The listing builds one solid part. Answer for the finished solid, in the listing's coordinates (mm). Face numbers are marked on the shaded views. A direction names the side the tool comes from. Round coordinates to 2 decimals unless told otherwise and drop trailing zeros. Order: outer loops, then holes, each group sorted by start corner. A loop starts at its lowest first (then second) coordinate and runs counter-clockwise, first axis right, second up. Notation, with made-up numbers: (-32, 86.5) - (27, 86.5) arc R18 ccw to (27, 101.5) - close; hole circle Ø3 at (69.25, 83.5). An arc over 180 degrees is marked (long way). Use CSV: the item, a comma, the result in double quotes. Start each with the question number.
Item 1: Flat-ended cylindrical pins translate along their axes: P1, Ø24, axis at x = 1, y = -3, coming from the +Z side; P2, Ø8, axis at x = 7, y = 8.5, coming from the +Z side; P3, Ø3, axis at y = 2, z = 14.5, coming from the +X side. Find the tip coordinate at first contact, or state that the pin passes through.
Item 2: For the marked faces 4 and 5, determine the directions among +Z, -Z, +X, -X, +Y, -Y from which every point of the face is accessible in a straight line to the end or side of a thin tool.
Item 3: Straight lines are drawn through the part: line 1 along Y through (x, z) = (0, 42.45); line 2 along Z through (x, y) = (2.5, 7); line 3 along Z through (x, y) = (-12.5, -3). For each, find the intervals that lie inside material, in ascending order. Write a range as [from, to].
Item 4: Find section D-D, the plane z = 50. Give the vertices of the cut face in (x, y).
Item 5: Determine the mould class of the marked faces 1, 2 and 3 for opening direction Z: +Z half, -Z half, draft (parallel to the pull), parting line (faces both ways), or undercut.
Solid Edge part; units mm, degrees
sketch "Sketch1" plane through (0, 0, 0) normal (0, 0, 1) x (1, 0, 0)
  line L0 (-20.5, -20.5) -> (20.5, -20.5)
  line L1 (20.5, -20.5) -> (20.5, 20.5)
  line L2 (20.5, 20.5) -> (-20.5, 20.5)
  line L3 (-20.5, 20.5) -> (-20.5, -20.5)
extrude "ProtrusiónExtruida_1" add sketch "Sketch1" along normal blind 41
sketch "Sketch2" plane through (0, 0, 41) normal (0, 0, 1) x (1, 0, 0)
  circle A0 centre (0, 0) radius 9
  circle A1 centre (0, 0) radius 11
extrude "ProtrusiónExtruida_2" add sketch "Sketch2" along normal blind 2
sketch "Sketch3" plane through (0, 0, 41) normal (0, 0, 1) x (1, 0, 0)
  circle A0 centre (0, 0) radius 2.5
extrude "ProtrusiónExtruida_3" add sketch "Sketch3" along normal blind 20
sketch "Sketch4" plane through (0, 0, 0) normal (0, -1, 0) x (1, 0, 0)
  line L0 (2.5, 58) -> (8, 58)
  line L1 (8, 58) -> (8, 57)
  line L2 (8, 57) -> (6, 57)
  line L3 (6, 57) -> (6, 45)
  line L4 (6, 45) -> (2.5, 45)
  line L5 (2.5, 45) -> (2.5, 58)
revolve "RevolvedProtrusion1" add sketch "Sketch4" angle 360 about axis through (0, 0, -54) along (0, 0, 1)
sketch "Sketch5" plane through (20.5, 0, 20.5) normal (1, 0, 0) x (0, 1, 0)
  line L0 (20.5, -11.5) -> (20.5, 13)
  line L1 (20.5, 13) -> (20.49, 13)
  line L2 (20.49, 13) -> (20.49, -11.5)
  line L3 (20.49, -11.5) -> (20.5, -11.5)
extrude "Cutout1" cut sketch "Sketch5" against normal up to next
sketch "Sketch6" plane through (0, 20.49, 21.25) normal (0, 1, 0) x (-1, 0, 0)
  line L0 (20.5, 12.25) -> (20.5, -12.25)
  line L1 (20.49, -12.25) -> (20.5, -12.25)
  line L2 (20.49, 12.25) -> (20.49, -12.25)
  line L3 (20.5, 12.25) -> (20.49, 12.25)
extrude "Cutout2" cut sketch "Sketch6" against normal up to next
sketch "Sketch7" plane through (-20.49, -0.005, 21.25) normal (-1, 0, 0) x (0, -1, 0)
  line L0 (20.485, 12.25) -> (20.485, -12.25)
  line L1 (20.485, -12.25) -> (20.495, -12.25)
  line L2 (20.495, -12.25) -> (20.495, 12.25)
  line L3 (20.495, 12.25) -> (20.485, 12.25)
extrude "Cutout3" cut sketch "Sketch7" against normal up to next
sketch "Sketch8" plane through (0.005, -20.49, 21.25) normal (0, -1, 0) x (1, 0, 0)
  line L0 (20.485, 12.25) -> (20.485, -12.25)
  line L1 (20.485, -12.25) -> (20.495, -12.25)
  line L2 (20.495, 12.25) -> (20.495, -12.25)
  line L3 (20.495, 12.25) -> (20.485, 12.25)
extrude "Cutout4" cut sketch "Sketch8" against normal up to next
fillet "Redondeo_1" [suppressed]
fillet "Redondeo_2" radius 3.5 4 edges at (20.49, -20.49, 21.25) (-20.49, -20.49, 21.25) (20.49, 20.49, 21.25) (-20.49, 20.49, 21.25)
fillet "Redondeo_3" radius 3.5 8 edges at (-20.5, 20.5, 37.25) (-20.5, -20.5, 37.25) (-20.5, 20.5, 4.5) (-20.5, -20.5, 4.5) (20.5, -20.5, 4.5) (20.5, -20.5, 37.25) (20.5, 20.5, 37.25) (20.5, 20.5, 4.5)
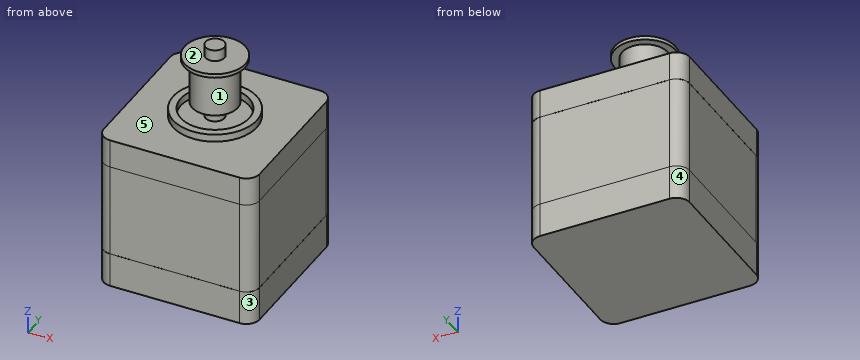
Worked out:
1,P1,"stops at z = 61"
1,P2,"stops at z = 58"
1,P3,"stops at x = 20.49"
2,face 4,"+Z, -Z, -X, +Y"
2,face 5,"+Z"
3,line 1,"y = [-11, -9], [-2.5, 2.5], [9, 11]"
3,line 2,"z = [0, 41], [57, 58]"
3,line 3,"z = [0, 41]"
4,outline,"circle Ø12 at (0, 0)"
5,face 1,"undercut"
5,face 2,"+Z half"
5,face 3,"draft"
